Autodesk Fusion 360 part; units mm, degrees
sketch "Sketch1" plane through (0, 0, 0) normal (0, 0, 1) x (1, 0, 0)
  line L0 (3.5355, 3.5355) -> (67.7657, 67.7657)
  line L1 (98.2899, 4.6985) -> (75.9997, 65.9403)
  line L2 (-3.5355, 3.5355) -> (-8.4853, 8.4853)
  arc A0 (75.9997, 65.9403) -> (67.7657, 67.7657) centre (71.3012, 64.2302) ccw
  line L3 (-8.4853, 12.7279) -> (-7.6674, 13.5458)
  line L4 (-10.6066, 10.6066) -> (-5.6066, 10.6066) construction
  arc A1 (-3.5355, 3.5355) -> (3.5355, 3.5355) centre (0, 7.0711) ccw
  arc A2 (-8.4853, 12.7279) -> (-8.4853, 8.4853) centre (-6.364, 10.6066) ccw
  line L5 (7.0711, 0) -> (43.5529, 36.4818)
  line L6 (93.5914, 2.9884) -> (84.7228, 27.3546)
  arc A3 (84.7228, 27.3546) -> (43.5529, 36.4818) centre (61.2305, 18.8041) ccw
  circle A4 centre (69.2871, 55.145) radius 7.5
  arc A5 (0, -2.9289) -> (7.0711, 0) centre (0, 7.0711) ccw
  line L7 (0, -2.9289) -> (0, -2.9289)
  line L8 (-9.9476, 15.0524) -> (-10, 15)
  line L9 (-9.405, 14.8257) -> (-7.8804, 14.3792)
  arc A6 (-8.6295, -0.1981) -> (0, -2.9289) centre (0, 12.0711) ccw
  arc A7 (-10.4427, 14.5199) -> (-8.6295, -0.1981) centre (-2.8765, 7.9814) ccw
  arc A8 (-9.405, 14.8257) -> (-10.4427, 14.5199) centre (-9.6861, 13.866) ccw
  arc A9 (-7.6674, 13.5458) -> (-7.8804, 14.3792) centre (-8.021, 13.8993) ccw
  arc A10 (111.0144, 2.9071) -> (113.1357, 6.5813) centre (110.2379, 5.8048) ccw
  line L10 (97.9588, -2.7353) -> (97.9588, -2.7353)
  arc A11 (98.2899, 4.6985) -> (104.3967, 1.1339) centre (103.1256, 5.9696) ccw
  line L11 (115.5643, 7.8632) -> (115.5835, 7.7916)
  arc A12 (113.4375, 8.3138) -> (112.8363, 7.6985) centre (113.3193, 7.8279) ccw
  line L12 (104.3967, 1.1339) -> (111.0144, 2.9071)
  arc A13 (115.7269, 7.1545) -> (114.9811, 7.9382) centre (114.7447, 6.9665) ccw
  line L13 (113.1357, 6.5813) -> (112.8363, 7.6985)
  arc A14 (106.7976, -4.6851) -> (115.7269, 7.1545) centre (105.9051, 5.275) ccw
  line L14 (114.9811, 7.9382) -> (113.4375, 8.3138)
  arc A15 (93.5914, 2.9884) -> (97.9588, -2.7353) centre (103.1064, 5.7205) ccw
  arc A16 (97.9588, -2.7353) -> (106.7976, -4.6851) centre (105.4588, 10.2551) ccw
  point P0 (100, 0)
  point P1 (-7.0711, 14.1421)
  point P2 (95.6559, -0.9674)
  point P3 (102.727, -0.9674)
  point P4 (99.4233, -0.1988)
  point P5 (112.6181, 8.5131)
  dimension "d2" = 100
  dimension "d6" = 15
  dimension "d9" = 5
  dimension "d10" = 45
  dimension "d11" = 5
  dimension "d13" = 5
  dimension "d15" = 3
  dimension "d19" = 25
  dimension "d20" = 15
  dimension "d21" = 10
  dimension "d23" = 10
  dimension "d26" = 15
  dimension "d27" = 10
  dimension "d28" = 1
  dimension "d29" = 0.5
extrude "Extrude1" add sketch "Sketch1" along normal blind 100
sketch "Sketch2" plane through (0, 0, 0) normal (-0.7071, 0.7071, 0) x (-0.7071, -0.7071, 0)
  line L0 (-95.8352, 0) -> (-5, 0)
  line L1 (-5, 0) -> (-5, 100)
  line L2 (-5, 100) -> (-95.8352, 100)
  line L3 (-95.8352, 100) -> (-95.8352, 0)
  ellipse E0 centre (-30, 50) end of major axis (-30, 90) minor radius 20
  line L4 (-30, 10) -> (-30, 90)
  line L5 (-10, 50) -> (-50, 50)
sketch "Sketch3" plane through (88.3022, 32.1394, 0) normal (0.9397, 0.342, 0) x (-0.342, 0.9397, 0)
  line L0 (-29.202, 0) -> (35.9702, 0)
  line L1 (35.9702, 0) -> (35.9702, 100)
  line L2 (35.9702, 100) -> (-29.202, 100)
  line L3 (-29.202, 100) -> (-29.202, 0)
  ellipse E0 centre (-15, 50) end of major axis (-15, 90) minor radius 10
  line L4 (-15, 10) -> (-15, 90)
  line L5 (-5, 50) -> (-25, 50)
  dimension "d35" = 20
extrude "Extrude3" [suppressed]
extrude "Extrude4" [suppressed]
The listing builds one solid part. Answer for the finished solid, in the listing's coordinates (mm). A direction names the side the tool comes from. Give positions to 0.01 mm unless a question says otherwise; leave off trailing zeros. Write each loop counter-clockwise with the first axis right and the second up, starting at its lowest first coordinate (ties: lowest second). Pieces come first, ordered by that corner, then holes.
Item 1: Find the intervals of material crossed by line 1 along X through (y, z) = (7.5, 58.5); line 2 along X through (y, z) = (-1, 10); line 3 along X through (y, z) = (5.5, 27.5), in increasing order.
Item 2: Section D-D, the plane x = 45 is taken. Write down the section's boundary in (y, z).
Item 3: Determine the mould class of faces 1 (the cylindrical face through (95.27, -0.33, 49.3)), 2 (the flat face through (107.66, 2.01, 49.3)), 3 (the cylindrical face through (-9.364, 10.574, 49.3)) for opening direction Y: released by +Y, released by -Y, zero draft, split by the parting line, or undercut.
Item 4: Section B-B, the plane y = 11 is taken. Write down the section's boundary in (x, z).
Item 5: Section A-A, the plane y = 25.5 is taken. Write down the section's boundary in (x, z), plus the area to 3 significant figures.
Item 6: Flat-ended cylindrical pins translate along their axes: P1, Ø1.5, axis at x = 49.5, z = 10, coming from the +Y side; P2, Ø9, axis at x = 69.29, y = 55.14, coming from the +Z side; P3, Ø6, axis at x = 40, z = 15, coming from the -Y side; P4, Ø8, axis at x = 9, z = 26, coming from the +Y side. Find the tip coordinate at first contact, or state that the pin passes through.
Item 7: Section C-C, the plane z = 42.5 is taken. Write down the section's boundary in (x, y) (1 decimal).
Item 8: Which of the six approach directions +Z, -Z, +X, -X, +Y, -Y give full straight-line access (tool end or side, diameter ignored) to faces 4 (the flat face through (-6, 6, 49)), 5 (the flat face through (25.06, 17.99, 49.3)), 6 (the flat face through (51, 43, 0)), 7 (the flat face through (51, 43, 100)), 8 (the flat face through (35, 35, 49))?
Completed:
1. line 1: x = -12.86 to -7.5, 7.5 to 14.57, 91.95 to 97.27, 112.89 to 115.59
1. line 2: x = -7.36 to 5.9, 95.84 to 113.69
1. line 3: x = -12.56 to -5.5, 5.5 to 12.57, 92.68 to 98, 113.22 to 115.9
2. outline: (37.82, 0) - (45, 0) - (45, 100) - (37.82, 100) - close
3. face 1: released by -Y
3. face 2: released by +Y
3. face 3: undercut
4. outline: (-12.41, 0) - (-9.34, 0) - (-9.34, 100) - (-12.41, 100) - close; (11, 0) - (18.07, 0) - (18.07, 100) - (11, 100) - close; (90.68, 0) - (96, 0) - (96, 100) - (90.68, 100) - close
5. outline: (25.5, 0) - (32.57, 0) - (32.57, 100) - (25.5, 100) - close; (85.4, 0) - (90.72, 0) - (90.72, 100) - (85.4, 100) - close
5. area: 1,240 mm2
6. P1: stops at y = 50.25
6. P2: passes through
6. P3: stops at y = 29.93
6. P4: stops at y = 13
7. outline: (-10.4, 14.5) arc R10 ccw to (-8.6, -0.2) arc R15 ccw to (0, -2.9) arc R10 ccw to (7.1, 0) - (43.6, 36.5) arc R25 cw to (84.7, 27.4) - (93.6, 3) arc R9.9 ccw to (98, -2.7) arc R15 ccw to (106.8, -4.7) arc R10 ccw to (115.7, 7.2) arc R1 ccw to (115, 7.9) - (113.4, 8.3) arc R0.5 ccw to (112.8, 7.7) - (113.1, 6.6) arc R3 cw to (111, 2.9) - (104.4, 1.1) arc R5 cw to (98.3, 4.7) - (76, 65.9) arc R5 ccw to (67.8, 67.8) - (3.5, 3.5) arc R5 cw to (-3.5, 3.5) - (-8.5, 8.5) arc R3 cw to (-8.5, 12.7) - (-7.7, 13.5) arc R0.5 ccw to (-7.9, 14.4) - (-9.4, 14.8) arc R1 ccw to start; hole circle Ø15 at (69.3, 55.1)
8. face 4: +Z, -Z
8. face 5: +Z, -Z, -Y
8. face 6: -Z, +X, -X, +Y, -Y
8. face 7: +Z, +X, -X, +Y, -Y
8. face 8: +Z, -Z, +Y
